Part model, mm, in its own coordinate system. Give positions to 0.01 mm unless a question says otherwise; leave off trailing zeros. Write each loop counter-clockwise with the first axis right and the second up, starting at its lowest first coordinate (ties: lowest second). Pieces come first, ordered by that corner, then holes. Notation, with made-up numbers: M 0.5,78.5 L 13.5,78.5 A22 ccw 13.5,106.5 Z; hole C 40,-30.75 d5. An arc over 180 degrees is marked long. Use CSV: the item, a comma, the result in double quotes. Start each with the question number.
1. Band-saw the part on A-A, the plane y = 35. List the corners of the cut face in (x, z) (3 decimals).
2. Band-saw the part on B-B, the plane x = 10.75. List the corners of the cut face in (y, z) (3 decimals).
3. Drop a flat-ended pin along its axis: pin 1 Ø1 at (y, z) = (24, 292.5) entering from -X. Give the stop position or say it passes through.
4. Band-saw the part on C-C, the plane z = 300.5. List the corners of the cut face in (x, y) (3 decimals), then the cut area to 3 significant figures.
5. Drill centre lines: line 1 along X through (y, z) = (14, 697) (3 decimals); line 2 along Y through (x, z) = (9.75, 251) (3 decimals); line 3 along X through (y, z) = (3, 476.5). Where is each one in solid material? Low to high. Write a range as from..to.
Autodesk Inventor part; units mm, degrees
ref_plane "YZ Plane" through (0, 0, 0) normal (1, 0, 0) x (0, 1, 0)
ref_plane "XZ Plane" through (0, 0, 0) normal (0, 1, 0) x (-1, 0, 0)
ref_plane "XY Plane" through (0, 0, 0) normal (0, 0, 1) x (1, 0, 0)
sketch "Sketch1" plane through (0, 0, 0) normal (0, 0, 1) x (1, 0, 0)
  line L0 (3.175, 0) -> (22.225, 0)
  line L1 (25.4, 3.175) -> (25.4, 47.625)
  line L2 (22.225, 50.8) -> (3.175, 50.8)
  line L3 (0, 47.625) -> (0, 3.175)
  arc A0 (3.175, 50.8) -> (0, 47.625) centre (3.175, 47.625) ccw
  arc A1 (25.4, 47.625) -> (22.225, 50.8) centre (22.225, 47.625) ccw
  arc A2 (22.225, 0) -> (25.4, 3.175) centre (22.225, 3.175) ccw
  arc A3 (0, 3.175) -> (3.175, 0) centre (3.175, 3.175) ccw
  line L4 (6.35, 47.625) -> (19.05, 47.625)
  line L5 (22.225, 44.45) -> (22.225, 6.35)
  line L6 (19.05, 3.175) -> (6.35, 3.175)
  line L7 (3.175, 6.35) -> (3.175, 44.45)
  arc A4 (6.35, 47.625) -> (3.175, 44.45) centre (6.35, 44.45) ccw
  arc A5 (22.225, 44.45) -> (19.05, 47.625) centre (19.05, 44.45) ccw
  arc A6 (3.175, 6.35) -> (6.35, 3.175) centre (6.35, 6.35) ccw
  arc A7 (19.05, 3.175) -> (22.225, 6.35) centre (19.05, 6.35) ccw
  point P0 (0, 0)
  point P1 (25.4, 0)
  point P2 (0, 50.8)
  dimension "d0" = 50.8
  dimension "d1" = 25.4
  dimension "d2" = 3.175
  dimension "d3" = 3.175
  dimension "d4" = 3.175
  dimension "d5" = 3.175
  dimension "d6" = 3.175
  dimension "d7" = 3.175
  dimension "d8" = 3.175
  dimension "d9" = 3.175
  dimension "d10" = 3.175
extrude "Extrusion1" add sketch "Sketch1" along normal blind 762
properties part number "O channel 30 inch" material "Steel, Alloy"
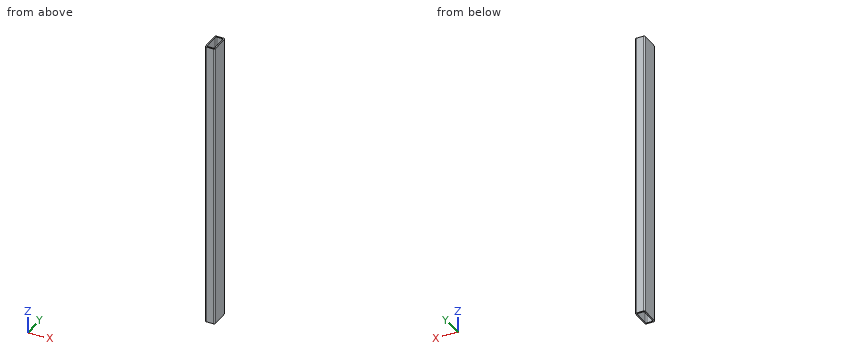
Output:
1,outline,"M 0,0 L 3.175,0 L 3.175,762 L 0,762 Z; M 22.225,0 L 25.4,0 L 25.4,762 L 22.225,762 Z"
2,outline,"M 0,0 L 3.175,0 L 3.175,762 L 0,762 Z; M 47.625,0 L 50.8,0 L 50.8,762 L 47.625,762 Z"
3,pin 1,"stops at x = 0"
4,outline,"M 0,3.175 A3.175 ccw 3.175,0 L 22.225,0 A3.175 ccw 25.4,3.175 L 25.4,47.625 A3.175 ccw 22.225,50.8 L 3.175,50.8 A3.175 ccw 0,47.625 Z; hole M 3.175,6.35 A3.175 ccw 6.35,3.175 L 19.05,3.175 A3.175 ccw 22.225,6.35 L 22.225,44.45 A3.175 ccw 19.05,47.625 L 6.35,47.625 A3.175 ccw 3.175,44.45 Z"
4,area,"444 mm²"
5,line 1,"x = 0..3.175, 22.225..25.4"
5,line 2,"y = 0..3.175, 47.625..50.8"
5,line 3,"x = 0..25.4"
